from build123d import *

# Parameters (mm, degrees)
SKIZZE1_R                       = 4
AUFSATZ_LINEAR_AUSTRAGEN1_DEPTH = 35
SKIZZE2_R                       = 2.5
SCHNITT_LINEAR_AUSTRAGEN1_DEPTH = 27
SKIZZE3_R                       = 12.769442974
SKIZZE3_R_2                     = 3
SCHNITT_LINEAR_AUSTRAGEN2_DEPTH = 30


with BuildPart() as part:
    # Skizze1 → Aufsatz-Linear austragen1 (new body)
    with BuildSketch(Plane.XY):
        with Locations((-21.202438913, 3.95852329)):
            Circle(SKIZZE1_R)
    extrude(amount=AUFSATZ_LINEAR_AUSTRAGEN1_DEPTH)

    # Skizze2 → Schnitt-Linear austragen1 (cut)
    with BuildSketch(Plane.XY.offset(35)):
        with Locations((-21.202438913, 3.95852329)):
            Circle(SKIZZE2_R)
    extrude(amount=-SCHNITT_LINEAR_AUSTRAGEN1_DEPTH, mode=Mode.SUBTRACT)

    # Skizze3 → Schnitt-Linear austragen2 (cut)
    with BuildSketch(Plane(origin=(0, 0, 0), x_dir=(-1, 0, 0), z_dir=(0, 0, -1))):
        with Locations((21.202438913, 3.95852329)):
            Circle(SKIZZE3_R)
        with Locations((21.202438913, 3.95852329)):
            Circle(SKIZZE3_R_2, mode=Mode.SUBTRACT)
    extrude(amount=-SCHNITT_LINEAR_AUSTRAGEN2_DEPTH, mode=Mode.SUBTRACT)


solid = part.part
Input: part model. Units: mm. Frame: model coordinates. A direction names the side the tool comes from. Round coordinates to 2 decimals unless told otherwise and drop trailing zeros. Order: outer loops, then holes, each group sorted by start corner. A loop starts at its lowest first (then second) coordinate and runs counter-clockwise, first axis right, second up.
1. Cut plane B-B, the plane y = 4.5. Output: boundary loops of the cut face in (x, z).
The answers:
outline: (-25.17, 30) - (-24.15, 30) - (-24.15, 0) - (-18.25, 0) - (-18.25, 30) - (-17.24, 30) - (-17.24, 35) - (-18.76, 35) - (-18.76, 8) - (-23.64, 8) - (-23.64, 35) - (-25.17, 35) - close
2. Mould query, pull axis X, two halves, no side actions, for faces 1 (the face through (-18.893, 3.001, 21.689)), 2 (the face through (-23, 7, 30)), 3 (the face through (-24.377, 1.525, 32.465)), 4 (the face through (-21, 4, 8)). Classes: released by +X, released by -X, zero draft, split by the parting line, or undercut.
The answers:
face 1: undercut
face 2: zero draft
face 3: split by the parting line
face 4: undercut
3. Cut plane D-D, the plane z = 6. Output: boundary loops of the cut face in (x, y).
The answers:
outline: circle Ø6 at (-21.2, 3.96)
4. Material intervals for line 1 (Z direction, x = -22, y = 0.75); line 2 (Z direction, x = -23.25, y = 5.25); line 3 (Y direction, x = -22.25, z = 24), sorted ascending.
The answers:
line 1: z = 30 to 35
line 2: z = 0 to 8
line 3: y = 1.15 to 1.69, 6.23 to 6.77
5. Set-up query: faces 5 (the face through (-18.822, 2.133, 14.79)), 6 (the face through (-23, 2, 35)). Return all of +Z, -Z, +X, -X, +Y, -Y with unobstructed straight access to the full face (end or side cutting, diameter ignored); none if empty.
The answers:
face 5: -Z
face 6: +Z, +X, -X, +Y, -Y
6. Cut plane A-A, the plane x = -20.5. Output: boundary loops of the cut face in (y, z), then the cut area to 3 significant figures.
The answers:
outline: (0.02, 30) - (1.04, 30) - (1.04, 0) - (6.88, 0) - (6.88, 30) - (7.9, 30) - (7.9, 35) - (6.36, 35) - (6.36, 8) - (1.56, 8) - (1.56, 35) - (0.02, 35) - close
area: 84.8 mm2
7. Cut plane C-C, the plane z = 19. Output: boundary loops of the cut face in (x, y).
The answers:
outline: circle Ø6 at (-21.2, 3.96); hole circle Ø5 at (-21.2, 3.96)
8. Pin query (flat end, axial travel): P1, Ø4, axis at x = -23.5, z = 29.5, coming from the +Y side; P2, Ø2.5, axis at x = -21, y = 3, coming from the +Z side; P3, Ø4, axis at x = -23.5, z = 16, coming from the -Y side. Return the tip coordinate at first contact, or that it passes through.
The answers:
P1: stops at y = 7.94
P2: stops at z = 8
P3: stops at y = 0.97
